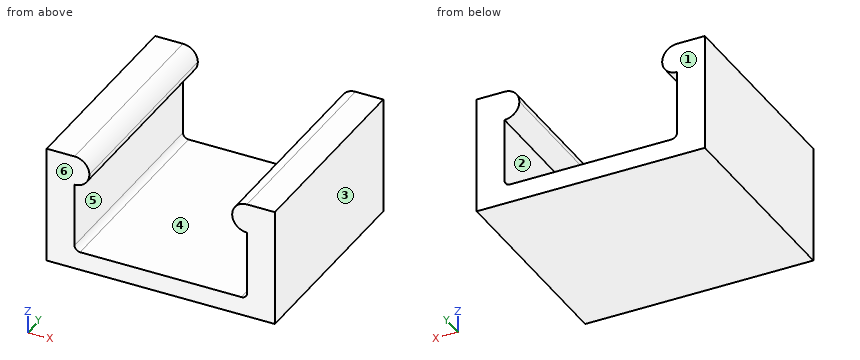
```python
from build123d import *

# Parameters (mm, degrees)
SKETCH_1_W          = 12.3
SKETCH_1_H          = 11.3
EXTRUDE_1_DEPTH     = 2
SKETCH_2_W          = 1.5
SKETCH_2_H          = 11.3
EXTRUDE_2_DEPTH     = 4.35
SKETCH_5_W          = 9.3
SKETCH_5_H          = 11.5
CUT_EXTRUDE_1_DEPTH = 1
SKETCH_8_W          = 1.6
SKETCH_8_H          = 11.3
EXTRUDE_5_DEPTH     = 0.8
SKETCH_9_W          = 1.6
SKETCH_9_H          = 11.3
EXTRUDE_6_DEPTH     = 0.8
FILLET_7_R          = 0.8
FILLET_8_R          = 0.3


with BuildPart() as part:
    # 스케치1 → 보스-돌출1 (new body)
    with BuildSketch(Plane.XY):
        Rectangle(SKETCH_1_W, SKETCH_1_H)
    extrude(amount=EXTRUDE_1_DEPTH)

    # 스케치2 → 보스-돌출2 (add)
    with BuildSketch(Plane.XY.offset(2)):
        with Locations((-5.4, 0)):
            Rectangle(SKETCH_2_W, SKETCH_2_H)
        with Locations((5.4, 0)):
            Rectangle(SKETCH_2_W, SKETCH_2_H)
    extrude(amount=EXTRUDE_2_DEPTH)

    # 스케치5 → 컷-돌출1 (cut)
    with BuildSketch(Plane.XY.offset(2)):
        Rectangle(SKETCH_5_W, SKETCH_5_H)
    extrude(amount=-CUT_EXTRUDE_1_DEPTH, mode=Mode.SUBTRACT)

    # 스케치8 → 보스-돌출5 (add)
    with BuildSketch(Plane(origin=(-4.65, 0, 0), x_dir=(0, 0, -1), z_dir=(1, 0, 0))):
        with Locations((-5.55, 0)):
            Rectangle(SKETCH_8_W, SKETCH_8_H)
    extrude(amount=EXTRUDE_5_DEPTH)

    # 스케치9 → 보스-돌출6 (add)
    with BuildSketch(Plane.ZY.offset(-4.65)):
        with Locations((5.55, 0)):
            Rectangle(SKETCH_9_W, SKETCH_9_H)
    extrude(amount=EXTRUDE_6_DEPTH)

    # 필렛7
    fillet_7_edges = [part.edges().sort_by_distance(p)[0] for p in [
        (3.85, 0, 6.35),
        (-3.85, 0, 6.35),
        (3.85, 0, 4.75),
        (-3.85, 0, 4.75),
    ]]
    fillet(fillet_7_edges, radius=FILLET_7_R - 0.0001)  # a hair under: the kernel refuses the full size

    # 필렛8
    fillet_8_edges = [part.edges().sort_by_distance(p)[0] for p in [
        (4.65, 0, 1),
        (-4.65, 0, 1),
    ]]
    fillet(fillet_8_edges, radius=FILLET_8_R)


solid = part.part
```
Geometry check sheet. Reference: the model listing, model coordinates, mm. Face numbers are marked on the shaded views. A direction names the side the tool comes from. Coordinates: 2 decimals unless noted, no trailing zeros. Order: outer loops, then holes, each group sorted by start corner. A loop starts at its lowest first (then second) coordinate and runs counter-clockwise, first axis right, second up. Notation, with made-up numbers: (27, 26.25) - (75, 26.25) arc R26 cw to (75, 56.25) - close; hole circle Ø8 at (75.25, -8). An arc over 180 degrees is marked (long way). Use one line per item in the form item = value.
1. Section check A-A (z = 4). Record the boundary of the cut face in (x, y).
Here are the results:
outline = (-6.15, -5.65) - (-4.65, -5.65) - (-4.65, 5.65) - (-6.15, 5.65) - close; (4.65, -5.65) - (6.15, -5.65) - (6.15, 5.65) - (4.65, 5.65) - close
2. Draft check along X on the marked faces 3, 4, 5 and 6. Enter one of: pulls with the +X half, pulls with the -X half, needs draft (parallel to the pull), parting line crosses it, or undercut.
Here are the results:
face_3 = pulls with the +X half
face_4 = undercut
face_5 = undercut
face_6 = needs draft
3. Access from +Z, -Z, +X, -X, +Y, -Y to the whole of each face (thin tool, end or side, straight path). Record for the marked faces 1 and 2.
Here are the results:
face_1 = +Z, -Z, +X, -X, +Y
face_2 = +Y, -Y
4. Section check C-C (x = -4). Record the boundary of the cut face in (y, z), then the cut area to 3 significant figures.
Here are the results:
outline = (-5.65, 0) - (5.65, 0) - (5.65, 1) - (-5.65, 1) - close; (-5.65, 5.08) - (5.65, 5.08) - (5.65, 6.02) - (-5.65, 6.02) - close
area = 21.8 mm²
5. Section check D-D (x = -0.25). Record the boundary of the cut face in (y, z).
Here are the results:
outline = (-5.65, 0) - (5.65, 0) - (5.65, 1) - (-5.65, 1) - close
6. Scan lines: line 1 (X direction, y = -1, z = 1.5); line 2 (Z direction, x = -3.5, y = -0.75); line 3 (X direction, y = 3.25, z = 5). Record each from-to range of solid material in increasing order.
Here are the results:
line_1 = -6.15 to -4.65, 4.65 to 6.15
line_2 = 0 to 1
line_3 = -6.15 to -4.07, 4.07 to 6.15
